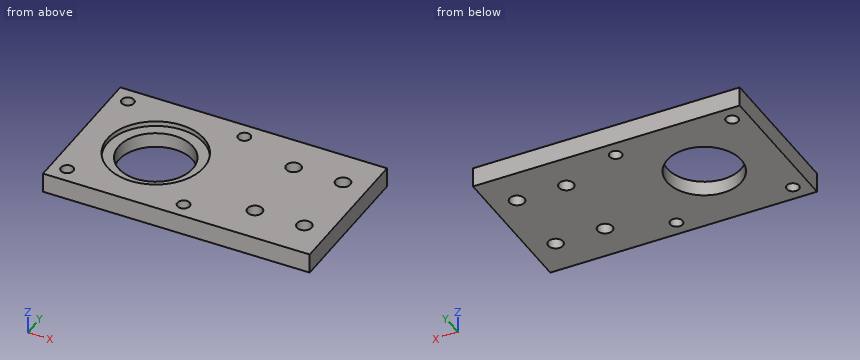
Autodesk Inventor part; units mm, degrees
ref_plane "YZ Plane" through (0, 0, 0) normal (1, 0, 0) x (0, 1, 0)
ref_plane "XZ Plane" through (0, 0, 0) normal (0, 1, 0) x (-1, 0, 0)
ref_plane "XY Plane" through (0, 0, 0) normal (0, 0, 1) x (1, 0, 0)
sketch "Szkic1" plane through (0, 0, 0) normal (0, 0, 1) x (1, 0, 0)
  circle A0 centre (30, 30) radius 15
  circle A1 centre (53.57, 6.43) radius 2.5
  circle A2 centre (6.43, 53.57) radius 2.5
  circle A3 centre (6.43, 6.43) radius 2.5
  circle A4 centre (53.57, 53.57) radius 2.5
  line L0 (0, 60) -> (0, 0)
  line L1 (0, 0) -> (78, 0)
  circle A5 centre (78, 45) radius 3
  circle A6 centre (98, 45) radius 3
  circle A7 centre (98, 15) radius 3
  circle A8 centre (78, 15) radius 3
  line L2 (108, 60) -> (108, 0)
  line L3 (0, 60) -> (108, 60)
  line L4 (108, 0) -> (78, 0)
  point P0 (35, 30)
  dimension "d12" = 6.43
  dimension "d13" = 6.43
  dimension "d14" = 47.14
  dimension "d15" = 47.14
  dimension "d16" = 30
  dimension "d17" = 10
  dimension "d18" = 10
  dimension "d19" = 30
  dimension "d20" = 30
  dimension "d21" = 108
extrude "Wyciągnięcie proste1" add sketch "Szkic1" along normal blind 8
thread "Gwint1"
thread "Gwint2"
thread "Gwint3"
thread "Gwint4"
sketch "Szkic2" plane through (0, 0, 8) normal (0, 0, 1) x (1, 0, 0)
  circle A0 centre (30, 30) radius 19.5
  circle A1 centre (53.57, 53.57) radius 2.5
  circle A2 centre (6.43, 6.43) radius 2.5
  circle A3 centre (6.43, 53.57) radius 2.5
  circle A4 centre (53.57, 6.43) radius 2.5
  line L0 (70, 60) -> (70, 0)
  line L1 (0, 60) -> (70, 60)
  line L2 (0, 0) -> (0, 60)
  line L3 (70, 0) -> (0, 0)
  circle A5 centre (30, 30) radius 15
  circle A6 centre (30, 30) radius 19.5
  circle A7 centre (30, 30) radius 15
  circle A8 centre (78, 15) radius 3
  circle A9 centre (98, 15) radius 3
  circle A10 centre (98, 45) radius 3
  circle A11 centre (78, 45) radius 3
  circle A12 centre (53.57, 53.57) radius 2.5
  circle A13 centre (6.43, 6.43) radius 2.5
  circle A14 centre (6.43, 53.57) radius 2.5
  circle A15 centre (53.57, 6.43) radius 2.5
  line L4 (0, 60) -> (0, 0)
  line L5 (0, 0) -> (108, 0)
  line L6 (108, 0) -> (108, 60)
  line L7 (108, 60) -> (0, 60)
  point P0 (35, 30)
extrude "Wyciągnięcie proste2" cut sketch "Szkic2" against normal blind 2 contours A0
properties part number "Uchwyt silnika krokowego osi Y - płaski"
Check sheet for the modelled part. Datum: model origin and axes. Units: mm. Round coordinates to 2 decimals unless told otherwise and drop trailing zeros. Order: outer loops, then holes, each group sorted by start corner. A loop starts at its lowest first (then second) coordinate and runs counter-clockwise, first axis right, second up. Notation, with made-up numbers: M -39.75,-24 L -23.75,-24 A25 ccw -23.75,10 Z; hole C -6,18 d9. An arc over 180 degrees is marked long. Answer in a Markdown table with one row per item.
(1) Material ranges on line 1 along Y through (x, z) = (98, 4.25); line 2 along Y through (x, z) = (53.57, 4); line 3 along X through (y, z) = (43, 2), recorded low to high. Write a range as from..to.
Findings:
| item | result |
|---|---|
| line 1 | y = 0..12, 18..42, 48..60 |
| line 2 | y = 0..3.93, 8.93..51.07, 56.07..60 |
| line 3 | x = 0..22.52, 37.48..75.76, 80.24..95.76, 100.24..108 |
(2) Section check D-D on x = 27. Record the boundary of the cut face in (y, z).
Findings:
| item | result |
|---|---|
| outline | M 0,0 L 15.3,0 L 15.3,6 L 10.73,6 L 10.73,8 L 0,8 Z; M 44.7,0 L 60,0 L 60,8 L 49.27,8 L 49.27,6 L 44.7,6 Z |
(3) Section check A-A on x = 98. Record the boundary of the cut face in (y, z), plus the area to 3 significant figures.
Findings:
| item | result |
|---|---|
| outline | M 0,0 L 12,0 L 12,8 L 0,8 Z; M 18,0 L 42,0 L 42,8 L 18,8 Z; M 48,0 L 60,0 L 60,8 L 48,8 Z |
| area | 384 mm^2 |
(4) Section check C-C on y = 53.57. Record the boundary of the cut face in (x, z).
Findings:
| item | result |
|---|---|
| outline | M 0,0 L 3.93,0 L 3.93,8 L 0,8 Z; M 8.93,0 L 51.07,0 L 51.07,8 L 8.93,8 Z; M 56.07,0 L 108,0 L 108,8 L 56.07,8 Z |
(5) Section check B-B on z = 3. Give the number of separate pieces and of enclosed holes in the cut face, plus the area to 3 significant figures.
Findings:
| item | result |
|---|---|
| separate pieces | 1 |
| enclosed holes | 9 |
| area | 5,580 mm^2 |
